Can you work these out from the model? Positions are in its coordinate system, mm. Face numbers are marked on the shaded views. Give positions to 0.01 mm unless a question says otherwise; leave off trailing zeros. Loops run counter-clockwise (first coordinate to the right, second up) from the corner with the lowest first, then second, coordinate; pieces in that order, holes last. Notation, with made-up numbers: (15.5, 7.5) - (54.5, 7.5) arc R36 cw to (54.5, 41.5) - close; hole circle Ø9 at (8, -6). An arc over 180 degrees is marked (long way). Answer as a JSON object with one key per item and string values.
```python
from build123d import *

# Parameters (mm, degrees)
SKETCH1_R           = 12.3
BOSS_EXTRUDE1_DEPTH = 3.5
SKETCH2_R           = 12.3
SKETCH2_R_2         = 6
BOSS_EXTRUDE2_DEPTH = 5
CHAMFER1_SIZE       = 5
CHAMFER1_SIZE2      = 2.886751346


with BuildPart() as part:
    # Sketch1 → Boss-Extrude1 (new body)
    with BuildSketch(Plane(origin=(0, 0, 0), x_dir=(1, 0, 0), z_dir=(0, 1, 0))):
        Circle(SKETCH1_R)
    extrude(amount=BOSS_EXTRUDE1_DEPTH)

    # Sketch2 → Boss-Extrude2 (add)
    with BuildSketch(Plane(origin=(0, 3.5, 0), x_dir=(1, 0, 0), z_dir=(0, 1, 0))):
        Circle(SKETCH2_R)
        Circle(SKETCH2_R_2, mode=Mode.SUBTRACT)
    extrude(amount=BOSS_EXTRUDE2_DEPTH)

    # Chamfer1
    chamfer1_edges = [part.edges().sort_by_distance(p)[0] for p in [
        (-12.3, 8.5, 0),
    ]]
    chamfer1_side = [part.faces().sort_by_distance(p)[0] for p in [
        (-12.3, 4.25, 0),
    ]]
    chamfer(chamfer1_edges, length=CHAMFER1_SIZE, length2=CHAMFER1_SIZE2, reference=chamfer1_side[0])


solid = part.part
```
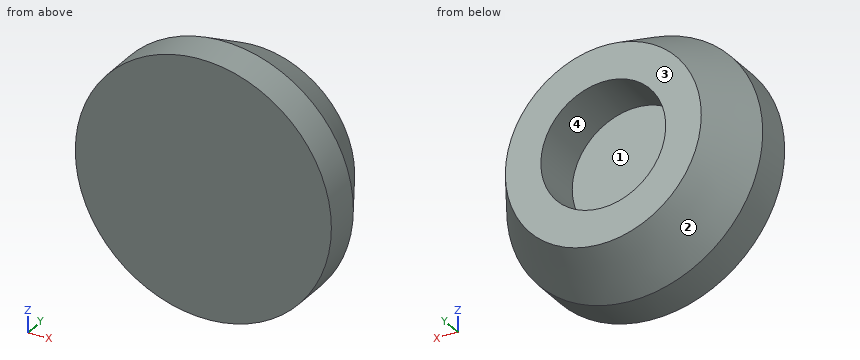
1) Imagine slicing it at B-B on x = 0. Write out the boundary of the cut face in (y, z), and give its area (3 significant figures).
Check sheet entries:
{"outline": "(0, -12.3) - (3.5, -12.3) - (8.5, -9.41) - (8.5, -6) - (3.5, -6) - (3.5, 6) - (8.5, 6) - (8.5, 9.41) - (3.5, 12.3) - (0, 12.3) - close", "area": "135 mm2"}
2) I'm going to push flat-ended pins straight in: P1, Ø5, axis at y = 2.5, z = -8.5, coming from the -X side; P2, Ø5, axis at y = 5, z = 5.5, coming from the +X side; P3, Ø4, axis at x = -3, y = 7, coming from the -Z side. Where does each tip first touch, or does it pass through?
Check sheet entries:
{"P1": "x = -10.74", "P2": "x = 11.79", "P3": "z = -11.13"}
3) Imagine slicing it at D-D on y = 2. Write out the boundary of the cut face in (x, z).
Check sheet entries:
{"outline": "circle Ø24.6 at (0, 0)"}
4) Imagine slicing it at C-C on y = 4.75. Write out the boundary of the cut face in (x, z).
Check sheet entries:
{"outline": "circle Ø23.16 at (0, 0); hole circle Ø12 at (0, 0)"}
5) If we mould it in two halves opening along Z, with no side actions, what happens to the marked faces 1, 2, 3 and 4? For each: released by +Z, released by -Z, zero draft, split by the parting line, or undercut.
Check sheet entries:
{"face 1": "undercut", "face 2": "split by the parting line", "face 3": "zero draft", "face 4": "undercut"}
6) I need wall thicknesses on L1, parallel to Y at x = 0.25, z = 1.25; L2, parallel to Z at x = 0, y = 5.95; L3, parallel to X at y = 5.45, z = 0. Which ranges of each line are inside material? Lowest first, please.
Check sheet entries:
{"L1": "0 to 3.5", "L2": "-10.89 to -6, 6 to 10.89", "L3": "-11.17 to -6, 6 to 11.17"}
7) Imagine slicing it at A-A on z = 0. Write out the boundary of the cut face in (x, y), and give its area (3 significant figures).
Check sheet entries:
{"outline": "(-12.3, 0) - (12.3, 0) - (12.3, 3.5) - (9.41, 8.5) - (6, 8.5) - (6, 3.5) - (-6, 3.5) - (-6, 8.5) - (-9.41, 8.5) - (-12.3, 3.5) - close", "area": "135 mm2"}
